For this review, take the finished solid that the model builds, in its own axes (mm). A direction names the side the tool comes from. Coordinates: 2 decimals unless noted, no trailing zeros. Write each loop counter-clockwise with the first axis right and the second up, starting at its lowest first coordinate (ties: lowest second). Pieces come first, ordered by that corner, then holes. Notation, with made-up numbers: (10.25, -37) - (41.25, -37) arc R30 cw to (41.25, -14) - close; hole circle Ø4 at (-28, 60). An arc over 180 degrees is marked (long way). Use one line per item in the form item = value. Start each with the question number.
1) Insertion check: P1, Ø1.5, axis at x = -11, z = 10, coming from the -Y side; P2, Ø1, axis at x = 7, y = 29, coming from the -Z side; P3, Ø2, axis at y = 85, z = 8.5, coming from the +X side. Each pin has a flat end and moves straight along its axis. Give the tip position at first contact, or say it passes through.
2) We need section D-D (z = -9). Give the boundary of the cut face in (x, y).
3) We need section A-A (z = 0). Give the boundary of the cut face in (x, y), plus the area to 3 significant figures.
4) We need section C-C (y = 12). Give the boundary of the cut face in (x, z).
5) We need section B-B (x = 0). Give the boundary of the cut face in (y, z), plus the area to 3 significant figures.
6) Mouldability with a two-part tool opening along Y and no side actions: class faces 5 (the flat face through (0, 27, -11.18)), 6 (the flat face through (0, 150, 0)), 7 (the cylindrical face through (0.14, 16.957, 0.651)), 8 (the flat face through (0, 55, 13)) as pulls with the +Y half, pulls with the -Y half, needs draft (parallel to the pull), parting line crosses it, or undercut.
7) Tool access review of faces 1 (the flat face through (0, 27, 11.18)), 2 (the flat face through (-12, 54.494, 0)), 3 (the flat face through (0, 55, -13)), 4 (the flat face through (10, 28, 0)): name each direction out of +Z, -Z, +X, -X, +Y, -Y from which nothing blocks a thin tool from reaching the whole face with its end or side.
8) For L1, parallel to Y at x = -1, z = 3.25; L2, parallel to X at y = 92, z = 0.75; L3, parallel to Z at x = 0.5, y = 66, list the stretches that pass through material, from the lowest coordinate up. Write a range as from..to.
```python
from build123d import *

# Parameters (mm, degrees)
SKETCH2_R           = 15
BOSS_EXTRUDE1_DEPTH = 150
CUT_EXTRUDE1_START  = 10
SKETCH3_W           = 30
SKETCH3_H           = 108.98871412
CUT_EXTRUDE1_DEPTH  = 100
CUT_EXTRUDE2_START  = -10
SKETCH3_2_W         = 30
SKETCH3_2_H         = 108.98871412
CUT_EXTRUDE2_DEPTH  = 100
SKETCH4_R           = 5
CUT_EXTRUDE3_DEPTH  = 100
CUT_EXTRUDE4_DEPTH  = 55


with BuildPart() as part:
    # Sketch2 → Boss-Extrude1 (new body)
    with BuildSketch(Plane(origin=(0, 0, 0), x_dir=(1, 0, 0), z_dir=(0, 1, 0))):
        with Locations(Location((0, 0, 0), (0, 0, 270))):
            Circle(SKETCH2_R)
    extrude(amount=BOSS_EXTRUDE1_DEPTH)

    # Sketch3 → Cut-Extrude1 (cut)
    with BuildSketch(Plane(origin=(0, 0, 0), x_dir=(0, 0, -1), z_dir=(1, 0, 0)).offset(CUT_EXTRUDE1_START)):
        Rectangle(SKETCH3_W, SKETCH3_H)
    extrude(amount=CUT_EXTRUDE1_DEPTH, mode=Mode.SUBTRACT)

    # Sketch3_2 → Cut-Extrude2 (cut)
    with BuildSketch(Plane(origin=(0, 0, 0), x_dir=(0, 0, -1), z_dir=(1, 0, 0)).offset(CUT_EXTRUDE2_START)):
        Rectangle(SKETCH3_2_W, SKETCH3_2_H)
    extrude(amount=-CUT_EXTRUDE2_DEPTH, mode=Mode.SUBTRACT)

    # Sketch4 → Cut-Extrude3 (cut)
    with BuildSketch(Plane(origin=(10, 0, 0), x_dir=(0, 0, -1), z_dir=(1, 0, 0))):
        with Locations((0.000339887, 12)):
            Circle(SKETCH4_R)
    extrude(amount=-CUT_EXTRUDE3_DEPTH, mode=Mode.SUBTRACT)

    # Sketch5 → Cut-Extrude4 (cut)
    with BuildSketch(Plane.XZ):
        with BuildLine():
            Line((-10, 11.180339887), (10, 11.180339887))
            ThreePointArc((10, 11.180339887), (0, 15), (-10, 11.180339887))
        make_face()
        with BuildLine():
            Line((-10, -11.180339887), (10, -11.180339887))
            ThreePointArc((10, -11.180339887), (0, -15), (-10, -11.180339887))
        make_face()
    extrude(amount=-CUT_EXTRUDE4_DEPTH, mode=Mode.SUBTRACT)


solid = part.part
```
Determined:
q1.P1 = 54.49
q1.P2 = -11.18
q1.P3 = 12.99
q2.outline = (-12, 54.49) - (-10, 54.49) - (-10, 0) - (10, 0) - (10, 54.49) - (12, 54.49) - (12, 150) - (-12, 150) - close
q3.outline = (-15, 54.49) - (-10, 54.49) - (-10, 17) - (10, 17) - (10, 54.49) - (15, 54.49) - (15, 150) - (-15, 150) - close; (-10, 0) - (10, 0) - (10, 7) - (-10, 7) - close
q3.area = 3,760 mm²
q4.outline = (-10, -11.18) - (10, -11.18) - (10, -5) - (-10, -5) - close; (-10, 5) - (10, 5) - (10, 11.18) - (-10, 11.18) - close
q5.outline = (0, -11.18) - (55, -11.18) - (55, -15) - (150, -15) - (150, 15) - (55, 15) - (55, 11.18) - (0, 11.18) - close; hole circle Ø10 at (12, 0)
q5.area = 4,000 mm²
q6.face_5 = needs draft
q6.face_6 = pulls with the +Y half
q6.face_7 = undercut
q6.face_8 = pulls with the -Y half
q7.face_1 = +Z, +X, -X, -Y
q7.face_2 = +Z, -Z, -X, -Y
q7.face_3 = -Z, +X, -X, -Y
q7.face_4 = +Z, -Z, +X, -Y
q8.L1 = 0..8.2, 15.8..150
q8.L2 = -14.98..14.98
q8.L3 = -14.99..14.99
